For this review, use the dimensioned drawing (mm, ordinates from the lowest corner) and the shaded views. Give positions to 0.01 mm unless a question says otherwise; leave off trailing zeros. Loops run counter-clockwise (first coordinate to the right, second up) from the corner with the lowest first, then second, coordinate; pieces in that order, holes last. Notation, with made-up numbers: (-38.5, 74.25) - (-19.5, 74.25) arc R14 cw to (-19.5, 97.25) - close; hole circle Ø6 at (56, -8). An arc over 180 degrees is marked (long way). Put each result on its own line as item: value.
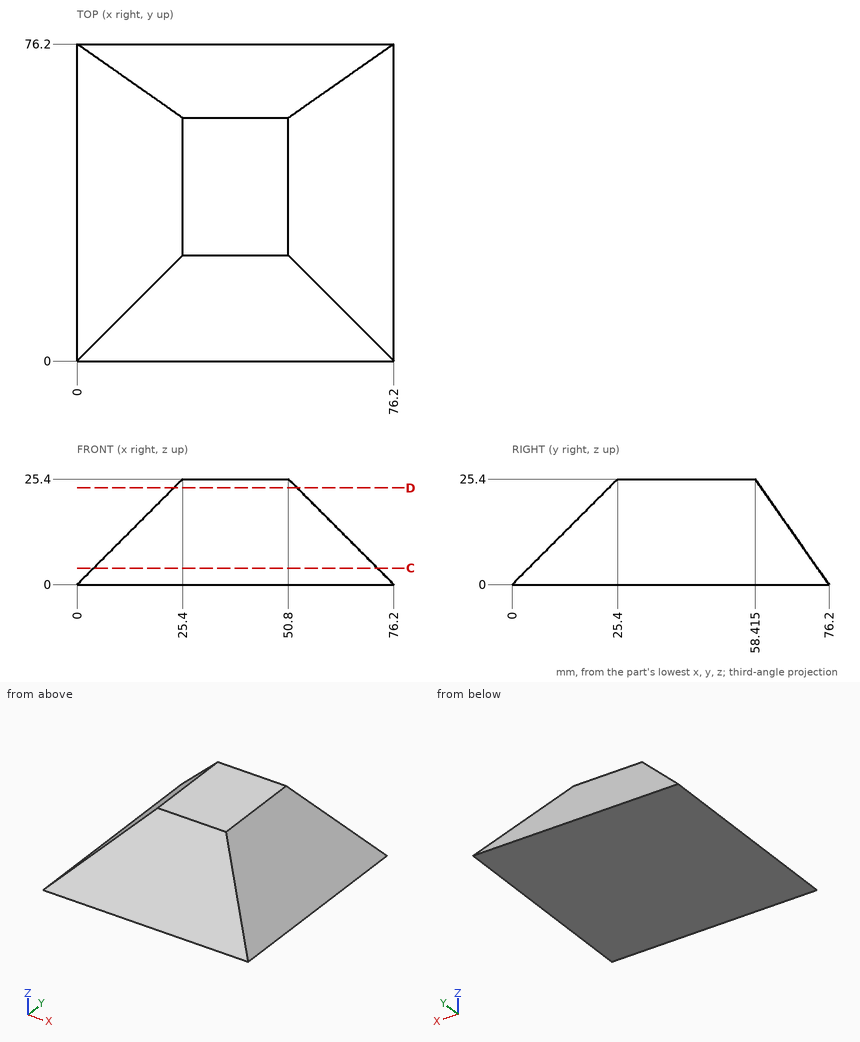
1) Take a section at C-C on z = 4. State the section outline as (x, y) points.
Geometry check:
outline: (4, 4) - (72.2, 4) - (72.2, 73.4) - (4, 73.4) - close
2) Take a section at D-D on z = 23.25. State the section outline as (x, y) points.
Geometry check:
outline: (23.25, 23.25) - (52.95, 23.25) - (52.95, 59.92) - (23.25, 59.92) - close
3) Insertion check: pin 1 Ø3 at (x, z) = (56, 3) entering from +Y; pin 2 Ø1.5 at (x, y) = (55, 40) entering from +Z; pin 3 Ø4 at (y, z) = (27, 19.5) entering from -X. Each pin has a flat end and moves straight along its axis. Give the tip position at first contact, or say it passes through.
Geometry check:
pin 1: stops at y = 75.15
pin 2: stops at z = 21.95
pin 3: stops at x = 17.5
4) Wall thickness on line 1 (Y direction, x = 51.5, z = 1.5); line 2 (X direction, y = 22, z = 19); line 3 (Y direction, x = 44, z = 18) (1 decimal): over which ranges is each line inside the solid? List them lowest first.
Geometry check:
line 1: y = 1.5 to 75.15
line 2: x = 19 to 57.2
line 3: y = 18 to 63.6
